Geometry check sheet. Reference: the model listing, model coordinates, mm. Face numbers are marked on the shaded views. A direction names the side the tool comes from. Round coordinates to 2 decimals unless told otherwise and drop trailing zeros. Write each loop counter-clockwise with the first axis right and the second up, starting at its lowest first coordinate (ties: lowest second). Pieces come first, ordered by that corner, then holes. Notation, with made-up numbers: (50.5, -23.5) - (109.5, -23.5) arc R11 cw to (109.5, -6.5) - close; hole circle Ø6 at (84, 50.5). An arc over 180 degrees is marked (long way). Return JSON: item names as keys, results as strings.
```python
from build123d import *

# Parameters (mm, degrees)
ESQUISSE1_W             = 27.85
ESQUISSE1_H             = 40
BOSS_EXTRU_1_DEPTH      = 6
ENL_V_START             = -3
ESQUISSE2_R             = 13.925
ENL_V_MAT_EXTRU_1_DEPTH = 3
ESQUISSE3_R             = 2.925
ENL_V_MAT_EXTRU_2_DEPTH = 10


with BuildPart() as part:
    # Esquisse1 → Boss.-Extru.1 (new body)
    with BuildSketch(Plane(origin=(0, 0, 0), x_dir=(0, 0, -1), z_dir=(1, 0, 0))):
        with Locations((-1.440517241, 18.893965517)):
            Rectangle(ESQUISSE1_W, ESQUISSE1_H)
        with BuildLine():
            ThreePointArc((12.484482759, -1.106034483), (-1.440517241, -15.031034483), (-15.365517241, -1.106034483))
            Line((-15.365517241, -1.106034483), (12.484482759, -1.106034483))
        make_face()
    extrude(amount=BOSS_EXTRU_1_DEPTH)

    # Esquisse2 → Enlèv. mat.-Extru.1 (cut)
    with BuildSketch(Plane(origin=(6, 0, 0), x_dir=(0, 0, -1), z_dir=(1, 0, 0)).offset(ENL_V_START)):
        with Locations((-1.440517241, -1.106034483)):
            Circle(ESQUISSE2_R)
    extrude(amount=ENL_V_MAT_EXTRU_1_DEPTH, mode=Mode.SUBTRACT)

    # Esquisse3 → Enlèv. mat.-Extru.2 (cut)
    with BuildSketch(Plane.ZY):
        with Locations((1.440517241, -1.106034483)):
            Circle(ESQUISSE3_R)
    extrude(amount=-ENL_V_MAT_EXTRU_2_DEPTH, mode=Mode.SUBTRACT)


solid = part.part
```
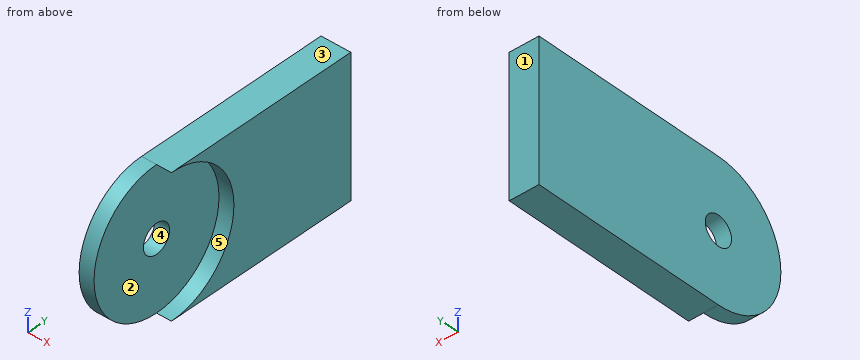
(1) Access from +Z, -Z, +X, -X, +Y, -Y to the whole of each face (thin tool, end or side, straight path). Record for the marked faces 4 and 5.
Response values:
{"face 4": "+X, -X", "face 5": "+X, -Y"}
(2) Section check B-B, the plane y = 9. Enter the section's corners in (x, z).
Response values:
{"outline": "(0, -12.48) - (6, -12.48) - (6, -8.14) - (3, -8.14) - (3, 11.02) - (6, 11.02) - (6, 15.37) - (0, 15.37) - close"}
(3) Gauge pin test, flat end, axial feed: pin 1 (1.5 mm diameter, centred on x = 5.5, z = 1.5, fed in from -Y). Record the tip position at first contact, or that the pin passes through.
Response values:
{"pin 1": "stops at y = 12.8"}
(4) Material ranges on line 1 along X through (y, z) = (5.5, 12.75); line 2 along Y through (x, z) = (3.1, -1.75); line 3 along Y through (x, z) = (1.3, -2), recorded low to high. Write a range as [from, to].
Response values:
{"line 1": "x = [0, 3]", "line 2": "y = [12.45, 38.89]", "line 3": "y = [-14.6, 38.89]"}
(5) Section check A-A, the plane x = 2.25. Enter the section's corners in (y, z) (3 decimals), plus the area to 3 significant figures.
Response values:
{"outline": "(-1.106, -12.484) - (38.894, -12.484) - (38.894, 15.366) - (-1.106, 15.366) arc R13.925 ccw to start; hole circle Ø5.85 at (-1.106, 1.441)", "area": "1,390 mm^2"}
(6) Release check for a two-part mould opening along Z. For the marked faces 1, 2 and 3 record: pulls with the +Z half, pulls with the -Z half, needs draft (parallel to the pull), parting line crosses it, or undercut.
Response values:
{"face 1": "needs draft", "face 2": "undercut", "face 3": "pulls with the +Z half"}
(7) Section check C-C, the plane z = -6.75. Enter the section's corners in (x, y).
Response values:
{"outline": "(0, -12.37) - (3, -12.37) - (3, 10.16) - (6, 10.16) - (6, 38.89) - (0, 38.89) - close"}
